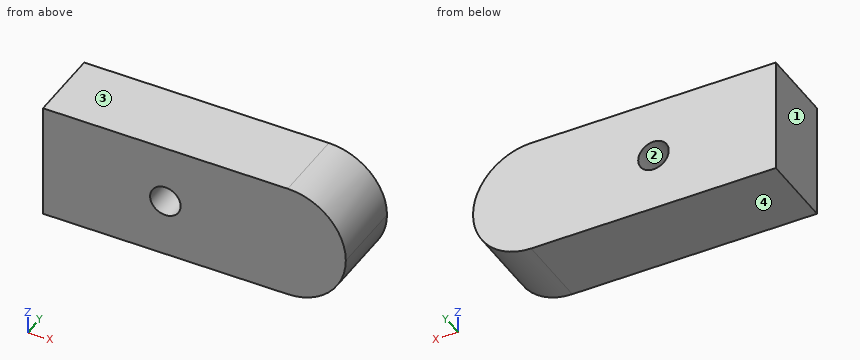
```python
from build123d import *

# Parameters (mm, degrees)
F0_R     = 5.1303996858
F1_DEPTH = 25.4


with BuildPart() as f1:
    # F0 (on Front) → F1 (new body)
    with BuildSketch(Plane.XZ):
        with BuildLine():
            ThreePointArc((41.0692058504, -19.5193476975), (21.5498581529, 0), (41.0692058504, 19.5193476975))
            Line((41.0692058504, 19.5193476975), (-41.0692058504, 19.5193476975))
            Line((-41.0692058504, 19.5193476975), (-41.0692058504, -19.5193476975))
            Line((-41.0692058504, -19.5193476975), (41.0692058504, -19.5193476975))
        make_face()
        Circle(F0_R, mode=Mode.SUBTRACT)
        with BuildLine():
            ThreePointArc((60.5885535479, 0), (54.8714689716, 13.8022631212), (41.0692058504, 19.5193476975))
            Line((41.0692058504, 19.5193476975), (41.0692058504, -19.5193476975))
            ThreePointArc((41.0692058504, -19.5193476975), (54.8714689716, -13.8022631212), (60.5885535479, 0))
        make_face()
        with BuildLine():
            Line((41.0692058504, -19.5193476975), (41.0692058504, 19.5193476975))
            ThreePointArc((41.0692058504, 19.5193476975), (21.5498581529, 0), (41.0692058504, -19.5193476975))
        make_face()
    extrude(amount=F1_DEPTH)


solid = f1.part
```
Check sheet for the modelled part. Datum: model origin and axes. Units: mm. Face numbers are marked on the shaded views. Coordinates: 2 decimals unless noted, no trailing zeros. Write each loop counter-clockwise with the first axis right and the second up, starting at its lowest first coordinate (ties: lowest second). Pieces come first, ordered by that corner, then holes. Notation, with made-up numbers: (39.5, 13.5) - (49.5, 13.5) arc R18 ccw to (49.5, 28.5) - close; hole circle Ø8 at (30, -25.5). An arc over 180 degrees is marked (long way). One line per question, with ' | ' between items.
Item 1: Sectioned sample at C-C on z = -2.5. Record the boundary of the cut face in (x, y), plus the area to 3 significant figures.
Determined:
outline: (-41.07, -25.4) - (-4.48, -25.4) - (-4.48, 0) - (-41.07, 0) - close; (4.48, -25.4) - (60.43, -25.4) - (60.43, 0) - (4.48, 0) - close | area: 2,350 mm2
Item 2: Thickness scan on line 1 (Z direction, x = 0, y = -17.25); line 2 (X direction, y = -10, z = -2); line 3 (X direction, y = -22, z = 1). Record the ranges inside material, lowest first. Write a range as [from, to].
Determined:
line 1: z = [-19.52, -5.13], [5.13, 19.52] | line 2: x = [-41.07, -4.72], [4.72, 60.49] | line 3: x = [-41.07, -5.03], [5.03, 60.56]
Item 3: Sectioned sample at B-B on y = -3.25. Record the boundary of the cut face in (x, z).
Determined:
outline: (-41.07, -19.52) - (41.07, -19.52) arc R19.52 ccw to (41.07, 19.52) - (-41.07, 19.52) - close; hole circle Ø10.26 at (0, 0)
Item 4: Mould release check, pull along Z, two halves, no side actions. Record for the marked faces 1, 2, 3 and 4: pulls with the +Z half, pulls with the -Z half, needs draft (parallel to the pull), parting line crosses it, or undercut.
Determined:
face 1: needs draft | face 2: undercut | face 3: pulls with the +Z half | face 4: pulls with the -Z half
Item 5: Sectioned sample at D-D on z = 17. Record the boundary of the cut face in (x, y).
Determined:
outline: (-41.07, -25.4) - (50.66, -25.4) - (50.66, 0) - (-41.07, 0) - close
Item 6: Sectioned sample at A-A on x = 0. Record the boundary of the cut face in (y, z).
Determined:
outline: (-25.4, -19.52) - (0, -19.52) - (0, -5.13) - (-25.4, -5.13) - close; (-25.4, 5.13) - (0, 5.13) - (0, 19.52) - (-25.4, 19.52) - close
Item 7: Gauge pin test, flat ends, axial feed: P1, Ø10, axis at y = -5.5, z = -10.5, coming from the +X side; P2, Ø5, axis at y = -11, z = -5, coming from the +X side. Record the tip position at first contact, or that the pin passes through.
Determined:
P1: stops at x = 59.8 | P2: stops at x = 60.43
